Work out the finished part from the listing and answer in its coordinate system (mm). A direction names the side the tool comes from. Coordinates: 2 decimals unless noted, no trailing zeros. Write each loop counter-clockwise with the first axis right and the second up, starting at its lowest first coordinate (ties: lowest second). Pieces come first, ordered by that corner, then holes. Notation, with made-up numbers: (8.25, 9) - (52.25, 9) arc R31 cw to (52.25, 43) - close; hole circle Ø5 at (40, 20.25). An arc over 180 degrees is marked (long way). Use a Markdown table: item, result. Add a question column.
(1) A tool of negligible diameter and unlimited length cuts with its end or side. For faces 1 (the face through (0, 296, 544)), 2 (the face through (-1141, 296, 150)), from which of +Z, -Z, +X, -X, +Y, -Y can it reach the whole face along a straight path? Write none if from no direction.
(2) Find the intervals of material crossed by line 1 (Z direction, x = -1393.5, y = 286); line 2 (Z direction, x = -123, y = 104), in increasing order. Write a range as from..to.
(3) Given pin 1 Ø4 at (x, y) = (-674.5, 174) entering from -Z; pin 2 Ø17.5 at (x, z) = (-2139.5, 57) entering from -Y; pin 3 Ø17.5 at (y, z) = (506, 79) entering from +X, each flat-ended and moving along its own axis, determine where each tip first touches the part or whether it passes through.
(4) The part is cut by section A-A, the plane x = -229. Give the vertices of the cut face in (y, z), then the cut area to 3 significant figures.
(5) The part is cut by section B-B, the plane y = 268.5. Give the vertices of the cut face in (x, z).
from build123d import *

# Parameters (mm, degrees)
F0_W     = 2250
F0_H     = 580
F1_DEPTH = 950
F2_W     = 1950
F2_H     = 150
F2_W_2   = 75
F3_DEPTH = 600
F4_W     = 40
F4_H     = 150
F4_W_2   = 350
F5_DEPTH = 2250
F6_SIZE  = 20


with BuildPart() as f1:
    # F0 (on Top) → F1 (new body)
    with BuildSketch(Plane.XY):
        with Locations((-1125, 290)):
            Rectangle(F0_W, F0_H)
    extrude(amount=F1_DEPTH)

    # F2 (on face) → F3 (cut)
    with BuildSketch(Plane.XZ):
        with Locations((-1125, 75)):
            Rectangle(F2_W, F2_H)
        with Locations((-2212.5, 75)):
            Rectangle(F2_W_2, F2_H)
        with Locations((-37.5, 75)):
            Rectangle(F2_W_2, F2_H)
    extrude(amount=-F3_DEPTH, mode=Mode.SUBTRACT)

    # F4 (on face) → F5 (cut)
    with BuildSketch(Plane(origin=(-2175, 0, 0), x_dir=(0, -1, 0), z_dir=(-1, 0, 0))):
        with Locations((-560, 75)):
            Rectangle(F4_W, F4_H)
        with Locations((-20, 75)):
            Rectangle(F4_W, F4_H)
        with Locations((-290, 75)):
            Rectangle(F4_W_2, F4_H)
    extrude(amount=-F5_DEPTH, mode=Mode.SUBTRACT)

    # F6
    f6_edges = [f1.edges().sort_by_distance(p)[0] for p in [
        (0, 0, 550),
        (-1125, 0, 150),
        (-2250, 0, 550),
        (-1125, 0, 950),
        (-2175, 40, 75),
        (-2100, 40, 75),
        (-2100, 115, 75),
        (-2175, 465, 75),
        (-2100, 465, 75),
        (-2100, 540, 75),
        (-2175, 540, 75),
        (-2175, 115, 75),
        (-75, 540, 75),
        (-75, 465, 75),
        (-75, 115, 75),
        (-75, 40, 75),
        (-150, 465, 75),
        (-150, 540, 75),
        (-150, 115, 75),
        (-150, 40, 75),
        (-112.5, 40, 0),
        (-75, 77.5, 0),
        (-112.5, 115, 0),
        (-150, 77.5, 0),
        (-112.5, 465, 0),
        (-75, 502.5, 0),
        (-112.5, 540, 0),
        (-150, 502.5, 0),
        (-2137.5, 465, 0),
        (-2175, 502.5, 0),
        (-2137.5, 540, 0),
        (-2100, 502.5, 0),
        (-2137.5, 115, 0),
        (-2137.5, 40, 0),
        (-2100, 77.5, 0),
        (-2175, 77.5, 0),
    ]]
    chamfer(f6_edges, length=F6_SIZE)


solid = f1.part
Model answer:
| question | item | result |
|---|---|---|
| 1 | face 1 | +Z, -Z, +X, +Y, -Y |
| 1 | face 2 | -Z |
| 2 | line 1 | 150..950 |
| 2 | line 2 | 9..950 |
| 3 | pin 1 | z = 150 |
| 3 | pin 2 | y = 40 |
| 3 | pin 3 | x = -75 |
| 4 | outline | (0, 170) - (20, 150) - (580, 150) - (580, 950) - (20, 950) - (0, 930) - close |
| 4 | area | 464,000 mm^2 |
| 5 | outline | (-2250, 150) - (0, 150) - (0, 950) - (-2250, 950) - close |
